from build123d import *

# Parameters (mm, degrees)
BOSS_EXTRUDE1_DEPTH          = 6.35
FILLET1_R                    = 10
M4X0_7_TAPPED_HOLE1_D        = 3.3
M4X0_7_TAPPED_HOLE2_D        = 3.3
FILLET2_R                    = 5
CUT_EXTRUDE1_DEPTH           = 111.566552356
CUT_EXTRUDE1_DEPTH_BACK      = 111.566552356
SKETCH10_R                   = 14.25
M3_CLEARANCE_HOLE1_OUTLINE_R = 1.7
M3_CLEARANCE_HOLE1_DEPTH     = 6.35


# Read off the part's stored shape, not the designer's step: M3 Clearance Hole1
with BuildPart() as part:
    # Sketch2 → Boss-Extrude1 (new body)
    with BuildSketch(Plane(origin=(0, 0, 0), x_dir=(1, 0, 0), z_dir=(0, 1, 0))):
        with BuildLine():
            Line((-36.071416662, -35.77), (-50.8, -35.77))
            Line((-50.8, -35.77), (-50.8, -98))
            Line((-50.8, -98), (-30.8, -98))
            Line((-30.8, -98), (-30.8, -48.47))
            Line((-30.8, -48.47), (-15.208520638, -48.47))
            ThreePointArc((-15.208520638, -48.47), (-26.414588628, -43.392505201), (-36.071416662, -35.77))
        make_face()
        with BuildLine():
            Line((0, -35.77), (-36.071416662, -35.77))
            ThreePointArc((-36.071416662, -35.77), (-26.414588628, -43.392505201), (-15.208520638, -48.47))
            Line((-15.208520638, -48.47), (0, -48.47))
            Line((0, -48.47), (0, -35.77))
        make_face()
        with BuildLine():
            Line((36.071416662, -35.77), (0, -35.77))
            Line((0, -35.77), (0, -48.47))
            Line((0, -48.47), (15.208520638, -48.47))
            ThreePointArc((15.208520638, -48.47), (26.414588628, -43.392505201), (36.071416662, -35.77))
        make_face()
        with BuildLine():
            Line((50.8, -98), (50.8, -35.77))
            Line((50.8, -35.77), (36.071416662, -35.77))
            ThreePointArc((36.071416662, -35.77), (26.414588628, -43.392505201), (15.208520638, -48.47))
            Line((15.208520638, -48.47), (30.8, -48.47))
            Line((30.8, -48.47), (30.8, -98))
            Line((30.8, -98), (50.8, -98))
        make_face()
        with BuildLine():
            Line((50.8, -35.77), (50.8, 0))
            ThreePointArc((50.8, 0), (46.973758453, -19.34182041), (36.071416662, -35.77))
            Line((36.071416662, -35.77), (50.8, -35.77))
        make_face()
        with BuildLine():
            Line((50.8, 0), (0, 0))
            Line((0, 0), (0, -35.77))
            Line((0, -35.77), (36.071416662, -35.77))
            ThreePointArc((36.071416662, -35.77), (46.973758453, -19.34182041), (50.8, 0))
        make_face()
        with BuildLine():
            ThreePointArc((50.8, 0), (0, 50.8), (-50.8, 0))
            Line((-50.8, 0), (0, 0))
            Line((0, 0), (50.8, 0))
        make_face()
        with BuildLine():
            Line((0, 0), (-50.8, 0))
            ThreePointArc((-50.8, 0), (-46.973758453, -19.34182041), (-36.071416662, -35.77))
            Line((-36.071416662, -35.77), (0, -35.77))
            Line((0, -35.77), (0, 0))
        make_face()
        with BuildLine():
            ThreePointArc((-36.071416662, -35.77), (-46.973758453, -19.34182041), (-50.8, 0))
            Line((-50.8, 0), (-50.8, -35.77))
            Line((-50.8, -35.77), (-36.071416662, -35.77))
        make_face()
    extrude(amount=BOSS_EXTRUDE1_DEPTH)

    # Fillet1
    fillet1_edges = [part.edges().sort_by_distance(p)[0] for p in [
        (30.8, 3.175, 48.47),
        (-30.8, 3.175, 48.47),
    ]]
    fillet(fillet1_edges, radius=FILLET1_R)

    # M4x0.7 Tapped Hole1 (through all)
    with Locations(Plane(origin=(0, 6.35, 0), x_dir=(1, 0, 0), z_dir=(0, 1, 0))):
        with Locations((-44.45, -46), (-44.45, -90), (44.45, -90), (44.45, -46)):
            Hole(M4X0_7_TAPPED_HOLE1_D / 2)

    # M4x0.7 Tapped Hole2 (through all)
    with Locations(Plane(origin=(0, 6.35, 0), x_dir=(1, 0, 0), z_dir=(0, 1, 0))):
        with Locations((-19.698321756, -40.903986603), (19.698321756, -40.903986603), (-44.261727213, -10.102450402), (-35.495149304, 28.306437004), (0, 45.4), (35.495149304, 28.306437004), (44.261727213, -10.102450402)):
            Hole(M4X0_7_TAPPED_HOLE2_D / 2)

    # Fillet2
    fillet2_edges = [part.edges().sort_by_distance(p)[0] for p in [
        (50.8, 3.175, 98),
        (30.8, 3.175, 98),
        (-30.8, 3.175, 98),
        (-50.8, 3.175, 98),
    ]]
    fillet(fillet2_edges, radius=FILLET2_R)

    # Sketch10 → Cut-Extrude1 (cut, two sides: drawn at the far end of the back side and taken through both)
    with BuildSketch(Plane(origin=(0, 6.35, 0), x_dir=(1, 0, 0), z_dir=(0, 1, 0)).offset(-CUT_EXTRUDE1_DEPTH_BACK)):
        with Locations(Location((0, 0, 0), (0, 0, 270))):
            Circle(SKETCH10_R)
    extrude(amount=CUT_EXTRUDE1_DEPTH + CUT_EXTRUDE1_DEPTH_BACK, mode=Mode.SUBTRACT)

    # M3 Clearance Hole1 outline → M3 Clearance Hole1 (cut)
    with BuildSketch(Plane(origin=(0, 0, 0), x_dir=(1, 0, 0), z_dir=(0, 1, 0))):
        with Locations((-20, 0)):
            Circle(M3_CLEARANCE_HOLE1_OUTLINE_R)
        with Locations((20, 0)):
            Circle(M3_CLEARANCE_HOLE1_OUTLINE_R)
        with Locations((0, 20)):
            Circle(M3_CLEARANCE_HOLE1_OUTLINE_R)
        with Locations((0, -20)):
            Circle(M3_CLEARANCE_HOLE1_OUTLINE_R)
    extrude(amount=M3_CLEARANCE_HOLE1_DEPTH, mode=Mode.SUBTRACT)


solid = part.part
The model under review builds one solid part; all positions refer to its coordinate system, in mm. A direction names the side the tool comes from. Coordinates: 2 decimals unless noted, no trailing zeros. Write each loop counter-clockwise with the first axis right and the second up, starting at its lowest first coordinate (ties: lowest second). Pieces come first, ordered by that corner, then holes. Notation, with made-up numbers: (26.5, 56.25) - (58.5, 56.25) arc R17 cw to (58.5, 72.25) - close; hole circle Ø4 at (-10.5, 83). An arc over 180 degrees is marked (long way). Answer as a JSON object with one key per item and string values. Group by question number.
1. Add section D-D (y = 1.25). Give the number of separate pieces and of enclosed holes in the cut face, plus the area to 3 significant figures.
2. Mouldability with a two-part tool opening along X and no side actions: class faces 1 (the face through (-43.046, 3.131, 8.987)), 2 (the face through (-49.3, 3.22, 96.57)), 3 (the face through (30.8, 3, 75)), 4 (the face through (50.8, 3, 47)) as pulls with the +X half, pulls with the -X half, needs draft (parallel to the pull), parting line crosses it, or undercut.
3. Clearance check with flat-ended pins moving along their axes: pin 1 Ø23 at (x, z) = (0, 0) entering from +Y; pin 2 Ø3 at (x, y) = (9.5, 3) entering from +Z. State where each tip first meets the part, or that it passes through.
4. Add section B-B (z = -20). Give the boundary of the cut face in (x, y), plus the area to 3 significant figures.
5. Add section A-A (x = 0). Give the boundary of the cut face in (y, z), plus the area to 3 significant figures.
6. Machinability: for faces 5 (the face through (-27.95, 3.22, 51.48)), 6 (the face through (45.91, 3.13, 10.03)), which of the approach directions +Z, -Z, +X, -X, +Y, -Y give a long, thin tool a straight path to every point of the face, cutting with its end or side? Answer none if there is none.
7. To check wall thickness, follow probe 1 along X at (y, z) = (4.5, 0); probe 2 along Z at (x, y) = (0, 2); probe 3 along Z at (x, y) = (21, 3.25). State the ranges of each line that lie inside material, in increasing order.
8. Add section C-C (z = 90). Give the boundary of the cut face in (x, y), plus the area to 3 significant figures.
Findings:
{
 "1": {"separate pieces": "1", "enclosed holes": "16", "area": "10,200 mm²"},
 "2": {"face 1": "undercut", "face 2": "pulls with the -X half", "face 3": "undercut", "face 4": "pulls with the +X half"},
 "3": {"pin 1": "through", "pin 2": "z = 48.47"},
 "4": {"outline": "(-46.7, 0) - (-1.7, 0) - (-1.7, 6.35) - (-46.7, 6.35) - close; (1.7, 0) - (46.7, 0) - (46.7, 6.35) - (1.7, 6.35) - close", "area": "571 mm²"},
 "5": {"outline": "(0, -50.8) - (6.35, -50.8) - (6.35, -47.05) - (0, -47.05) - close; (0, -43.75) - (6.35, -43.75) - (6.35, -21.7) - (0, -21.7) - close; (0, -18.3) - (6.35, -18.3) - (6.35, -14.25) - (0, -14.25) - close; (0, 14.25) - (6.35, 14.25) - (6.35, 18.3) - (0, 18.3) - close; (0, 21.7) - (6.35, 21.7) - (6.35, 48.47) - (0, 48.47) - close", "area": "385 mm²"},
 "6": {"face 5": "+Z, +Y, -Y", "face 6": "+Y, -Y"},
 "7": {"probe 1": "-50.8 to -21.7, -18.3 to -14.25, 14.25 to 18.3, 21.7 to 50.8", "probe 2": "-50.8 to -47.05, -43.75 to -21.7, -18.3 to -14.25, 14.25 to 18.3, 21.7 to 48.47", "probe 3": "-46.26 to -1.37, 1.37 to 39.89, 41.92 to 48.47"},
 "8": {"outline": "(-50.8, 0) - (-46.1, 0) - (-46.1, 6.35) - (-50.8, 6.35) - close; (-42.8, 0) - (-30.8, 0) - (-30.8, 6.35) - (-42.8, 6.35) - close; (30.8, 0) - (42.8, 0) - (42.8, 6.35) - (30.8, 6.35) - close; (46.1, 0) - (50.8, 0) - (50.8, 6.35) - (46.1, 6.35) - close", "area": "212 mm²"}
}
